Build history of the part. All positions in model axes, mm. Face numbers are marked on the shaded views. Round coordinates to 2 decimals unless told otherwise and drop trailing zeros. Write each loop counter-clockwise with the first axis right and the second up, starting at its lowest first coordinate (ties: lowest second). Pieces come first, ordered by that corner, then holes. Notation, with made-up numbers: M 2,-17.75 L 49,-17.75 A31 ccw 49,12.25 Z; hole C -12.5,36 d5. An arc over 180 degrees is marked long. Use a Markdown table: item, result.
Autodesk Fusion 360 part; units mm, degrees
sketch "Sketch1" plane through (0, 0, 0) normal (0, 1, 0) x (1, 0, 0)
  line L0 (0, 0) -> (11, 0)
  line L1 (11, 0) -> (11, -30)
  line L2 (11, -30) -> (0, -30)
  line L3 (0, -30) -> (0, 0)
  circle A0 centre (5.5, -15) radius 1.6
  circle A1 centre (5.5, -23) radius 2.5
  dimension "d1" = 30
  dimension "d2" = 11
  dimension "d3" = 3.2
  dimension "d4" = 5
  dimension "d5" = 15
  dimension "d6" = 8
  dimension "d7" = 5.5
extrude "Extrude1" add sketch "Sketch1" against normal blind 5 contours L0 L1 L2 L3 | A1
extrude "Extrude2" add sketch "Sketch1" against normal blind 2 from surface at -5 contours A1
fillet "Fillet1" radius 3 4 edges at (11, -2.5, 30) (0, -2.5, 30) (0, -2.5, 0) (11, -2.5, 0)
equation "d5 = d1 / 2"
equation "d7 = d2 / 2"
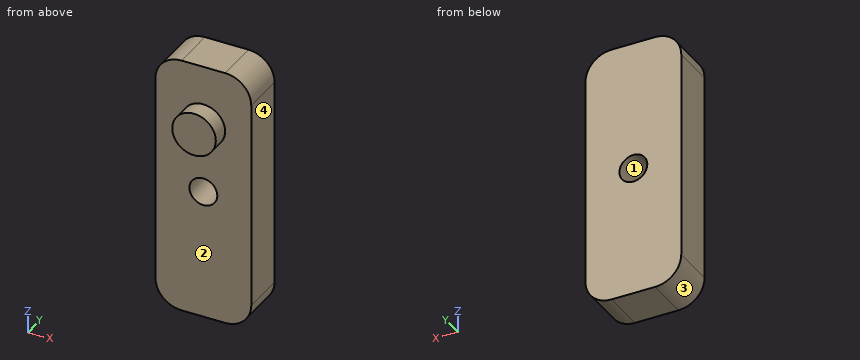
Q1. Cut at B-B on x = 5.5. Give the cut face in (y, z), and give its area (3 significant figures).
Response values:
| item | result |
|---|---|
| outline | M -7,20.5 L -5,20.5 L -5,16.6 L 0,16.6 L 0,30 L -5,30 L -5,25.5 L -7,25.5 Z; M -5,0 L 0,0 L 0,13.4 L -5,13.4 Z |
| area | 144 mm2 |
Q2. Cut at C-C on y = -3.75. Give the cut face in (x, z).
Response values:
| item | result |
|---|---|
| outline | M 0,3 A3 ccw 3,0 L 8,0 A3 ccw 11,3 L 11,27 A3 ccw 8,30 L 3,30 A3 ccw 0,27 Z; hole C 5.5,15 d3.2 |
Q3. Drill centre lines: L1, parallel to X at y = -1.85, z = 15; L2, parallel to Y at x = 0.5, z = 16.75; L3, parallel to Z at x = 5.5, y = -2.4. Where is each one in solid material? Low to high.
Response values:
| item | result |
|---|---|
| L1 | x = 0 to 3.9, 7.1 to 11 |
| L2 | y = -5 to 0 |
| L3 | z = 0 to 13.4, 16.6 to 30 |
Q4. Cut at D-D on z = 23. Give the cut face in (x, y).
Response values:
| item | result |
|---|---|
| outline | M 0,-5 L 3,-5 L 3,-7 L 8,-7 L 8,-5 L 11,-5 L 11,0 L 0,0 Z |
Q5. Drop a flat-ended pin along its axis: P1, Ø3.5, axis at x = 6, z = 10.5, coming from the -Y side. Give the stop position or say it passes through.
Response values:
| item | result |
|---|---|
| P1 | stops at y = -5 |
Q6. Cut at A-A on z = 15. Give the cut face in (x, y), and give its area (3 significant figures).
Response values:
| item | result |
|---|---|
| outline | M 0,-5 L 3.9,-5 L 3.9,0 L 0,0 Z; M 7.1,-5 L 11,-5 L 11,0 L 7.1,0 Z |
| area | 39.0 mm2 |
Q7. Two-plate mould, pull along X, no slides. Class the marked faces 1, 2, 3 and 4: +X half, -X half, draft (parallel to the pull), parting line (faces both ways), or undercut.
Response values:
| item | result |
|---|---|
| face 1 | undercut |
| face 2 | draft |
| face 3 | -X half |
| face 4 | +X half |
